Work out the finished part from the listing and answer in its coordinate system (mm). A direction names the side the tool comes from. Give positions to 0.01 mm unless a question says otherwise; leave off trailing zeros. Write each loop counter-clockwise with the first axis right and the second up, starting at its lowest first coordinate (ties: lowest second). Pieces come first, ordered by that corner, then holes. Notation, with made-up numbers: (-1.75, 0) - (4.25, 0) arc R12 cw to (4.25, 11) - close; hole circle Ø2 at (19.25, -34.5). An arc over 180 degrees is marked (long way). Write item = value, one per line.
from build123d import *

# Parameters (mm, degrees)
BOSS_EXTRUDE1_DEPTH = 20
SKETCH2_R           = 2.1
CUT_EXTRUDE1_DEPTH  = 8
SKETCH3_R           = 5
CUT_EXTRUDE2_DEPTH  = 3


with BuildPart() as part:
    # Sketch1 → Boss-Extrude1 (new body)
    with BuildSketch(Plane.XY):
        with BuildLine():
            Line((-8.366600265, -1.5), (8.366600265, -1.5))
            ThreePointArc((8.366600265, -1.5), (0, -8.5), (-8.366600265, -1.5))
        make_face()
    extrude(amount=BOSS_EXTRUDE1_DEPTH)

    # Sketch2 → Cut-Extrude1 (cut, through all)
    with BuildSketch(Plane(origin=(0, -1.5, 0), x_dir=(1, 0, 0), z_dir=(0, 1, 0))):
        with Locations((0, -10)):
            Circle(SKETCH2_R)
    extrude(amount=-CUT_EXTRUDE1_DEPTH, mode=Mode.SUBTRACT)

    # Sketch3 → Cut-Extrude2 (cut)
    with BuildSketch(Plane(origin=(0, -1.5, 0), x_dir=(1, 0, 0), z_dir=(0, 1, 0))):
        with Locations((0, -10)):
            Circle(SKETCH3_R)
    extrude(amount=-CUT_EXTRUDE2_DEPTH, mode=Mode.SUBTRACT)


solid = part.part
1. Find section D-D, the plane x = 4.25. Give the vertices of the cut face in (y, z).
Solution:
outline = (-7.36, 0) - (-1.5, 0) - (-1.5, 7.37) - (-4.5, 7.37) - (-4.5, 12.63) - (-1.5, 12.63) - (-1.5, 20) - (-7.36, 20) - close
2. Find section B-B, the plane z = 11. Give the vertices of the cut face in (x, y).
Solution:
outline = (-8.37, -1.5) arc R8.5 ccw to (-1.85, -8.3) - (-1.85, -4.5) - (-4.9, -4.5) - (-4.9, -1.5) - close; (1.85, -8.3) arc R8.5 ccw to (8.37, -1.5) - (4.9, -1.5) - (4.9, -4.5) - (1.85, -4.5) - close
3. For a pull along X with two mould halves and no side action, classify faces 1 (the flat face through (0, -4, 0)), 2 (the cylindrical face through (0.17, -8.5, 7.64)), 3 (the cylindrical face through (2.003, -6.476, 9.369)) as pulls with the +X half, pulls with the -X half, needs draft (parallel to the pull), parting line crosses it, or undercut.
Solution:
face_1 = needs draft
face_2 = parting line crosses it
face_3 = undercut
4. Find section C-C, the plane y = -4.75. Give the vertices of the cut face in (x, z), then the cut area to 3 significant figures.
Solution:
outline = (-7.05, 0) - (7.05, 0) - (7.05, 20) - (-7.05, 20) - close; hole circle Ø4.2 at (0, 10)
area = 268 mm^2
5. A tool of negligible diameter and unlimited length cuts with its end or side. For faces 4 (the cylindrical face through (-0.651, -2.979, 5.043)), 5 (the flat face through (0, -4, 20)), from which of +Z, -Z, +X, -X, +Y, -Y can it reach the whole face along a straight path? Write none if from no direction.
Solution:
face_4 = +Y
face_5 = +Z, +X, -X, +Y, -Y
6. Find section A-A, the plane x = 0. Give the vertices of the cut face in (y, z), then the cut area to 3 significant figures.
Solution:
outline = (-8.5, 0) - (-1.5, 0) - (-1.5, 5) - (-4.5, 5) - (-4.5, 7.9) - (-8.5, 7.9) - close; (-8.5, 12.1) - (-4.5, 12.1) - (-4.5, 15) - (-1.5, 15) - (-1.5, 20) - (-8.5, 20) - close
area = 93.2 mm^2
7. Given pin 1 (3 mm diameter, centred on y = -4.5, z = 12, fed in from +X); pin 2 (9 mm diameter, centred on x = 0, z = 10, fed in from -Y); pin 3 (3.5 mm diameter, centred on x = 0, z = 10, fed in from +Y); pin 4 (2 mm diameter, centred on y = -5.5, z = 7.5, fed in from +X), each flat-ended and moving along its own axis, determine where each tip first touches the part or whether it passes through.
Solution:
pin_1 = 7.95
pin_2 = -8.5
pin_3 = through
pin_4 = 7.21
8. Straight lines are drawn through the part: line 1 (Z direction, x = 0, y = -3.9); line 2 (Z direction, x = 0, y = -5.3); line 3 (X direction, y = -3.55, z = 10). For each, find the intervals that lie inside material, in ascending order.
Solution:
line_1 = 0 to 5, 15 to 20
line_2 = 0 to 7.9, 12.1 to 20
line_3 = -7.72 to -5, 5 to 7.72
